```python
from build123d import *

# Parameters (mm, degrees)
SKETCH1_W                    = 22
SKETCH1_H                    = 25
SKETCH1_R                    = 1.5
BASE_FLANGE1_DEPTH           = 1.5
EDGE_FLANGE1_STRIP_W         = 7.4732
EDGE_FLANGE1_STRIP_H         = 1.5
EDGE_FLANGE1_STRIP_CUT_DEPTH = 22
EDGE_FLANGE1_DEPTH           = 22
CUT_EXTRUDE1_DEPTH           = 10


# Sheet-metal steps are written as plain solids
with BuildPart() as part:
    # Sketch1 → Base-Flange1 (new body)
    with BuildSketch(Plane.XY):
        with Locations((0.834482759, -7.531034483)):
            Rectangle(SKETCH1_W, SKETCH1_H)
        with Locations((6.834482759, -13.834829283)):
            Circle(SKETCH1_R, mode=Mode.SUBTRACT)
        with Locations((-5.165517241, -13.834829283)):
            Circle(SKETCH1_R, mode=Mode.SUBTRACT)
        with Locations((-3.415517241, -1.662801421)):
            Circle(SKETCH1_R, mode=Mode.SUBTRACT)
        with Locations((4.994482759, -1.662801421)):
            Circle(SKETCH1_R, mode=Mode.SUBTRACT)
    extrude(amount=-BASE_FLANGE1_DEPTH)

    # Edge-Flange1 strip (across the edge) → Edge-Flange1 strip cut (cut)
    with BuildSketch(Plane(origin=(11.834482759, 4.968965517, 0), x_dir=(0, -1, 0), z_dir=(-1, 0, 0))):
        with Locations((-1.5, -0.75)):
            Rectangle(EDGE_FLANGE1_STRIP_W, EDGE_FLANGE1_STRIP_H)
    extrude(amount=EDGE_FLANGE1_STRIP_CUT_DEPTH, mode=Mode.SUBTRACT)

    # Edge-Flange1 section (across the edge) → Edge-Flange1 (add)
    with BuildSketch(Plane(origin=(11.834482759, 4.968965517, 0), x_dir=(0, -1, 0), z_dir=(-1, 0, 0))):
        with BuildLine():
            Line((0, 0.7366), (0, 14))
            Line((0, 14), (1.5, 14))
            Line((1.5, 14), (1.5, 0.7366))
            ThreePointArc((1.5, 0.7366), (1.715745145, 0.215745145), (2.2366, 0))
            Line((2.2366, 0), (2.2366, -1.5))
            ThreePointArc((2.2366, -1.5), (0.655084973, -0.844915027), (0, 0.7366))
        make_face()
    extrude(amount=EDGE_FLANGE1_DEPTH)

    # Sketch11 → Cut-Extrude1 (cut)
    with BuildSketch(Plane(origin=(0, 4.968965517, 0), x_dir=(1, 0, 0), z_dir=(0, 1, 0))):
        with BuildLine():
            Line((-4.050745128, -10.789495208), (-4.050745128, -4.789495208))
            ThreePointArc((-4.050745128, -4.789495208), (-5.800745128, -3.039495208), (-7.550745128, -4.789495208))
            Line((-7.550745128, -4.789495208), (-7.550745128, -10.789495208))
            ThreePointArc((-7.550745128, -10.789495208), (-5.800745128, -12.539495208), (-4.050745128, -10.789495208))
        make_face()
        with BuildLine():
            Line((8.840531004, -10.789495208), (8.840531004, -4.789495208))
            ThreePointArc((8.840531004, -4.789495208), (7.090531004, -3.039495208), (5.340531004, -4.789495208))
            Line((5.340531004, -4.789495208), (5.340531004, -10.789495208))
            ThreePointArc((5.340531004, -10.789495208), (7.090531004, -12.539495208), (8.840531004, -10.789495208))
        make_face()
    extrude(amount=-CUT_EXTRUDE1_DEPTH, mode=Mode.SUBTRACT)


solid = part.part
```
Could you check a few things on this model? Use its own coordinates, in mm. A direction names the side the tool comes from. Round coordinates to 2 decimals unless told otherwise and drop trailing zeros. Order: outer loops, then holes, each group sorted by start corner. A loop starts at its lowest first (then second) coordinate and runs counter-clockwise, first axis right, second up. Notation, with made-up numbers: M 53,38.25 L 104,38.25 A26 cw 104,59.25 Z; hole C 12.25,56 d3. An arc over 180 degrees is marked long. One line per question, with ' | ' between items. Start each with the question number.
(1) Please list where these lines run through material, in increasing order: line 1 along Z through (x, y) = (3.5, -7.25); line 2 along Y through (x, z) = (10.5, 10.75); line 3 along Z through (x, y) = (8.5, 3.25).
(2) Suppose I cut it at A-A on z = 9.75. List the corners of the cut face in (x, y) for me, then the cut area to 3 significant figures.
(3) Suppose I cut it at C-C on x = 4.5. List the corners of the cut face in (y, z) for me, then the cut area to 3 significant figures.
(4) For P1, Ø6.5, axis at x = -3.5, z = 8.5, coming from the -Y side; P2, Ø10, axis at x = -3.5, y = -2.5, coming from the -Z side; P3, Ø10, axis at x = -7, y = -5.5, coming from the +Z side, each with a flat end and sliding along its axis, tell me the tip position at first contact or that it passes through.
(5) For faces 4 (the face through (-5.76, 4.23, 3.04)), 5 (the face through (1, -8, 0)), 6 (the face through (0.99, 4.3, -0.86)), which set-ups out of +Z, -Z, +X, -X, +Y, -Y let a thin tool reach every point of the face, with its end or its side?
(6) Suppose I cut it at B-B on y = -0.5. List the corners of the cut face in (x, z) for me, then the cut area to 3 significant figures.
(7) Thinking about a two-plate mould opening in Y: for faces 1 (the face through (7.64, -12.57, -0.74)), 2 (the face through (1, -20.031, -1)), 3 (the face through (1, 4.969, 7)), which applies, +Y half, -Y half, draft (parallel to the pull), parting line (faces both ways), or undercut?
(8) Suppose I cut it at D-D on x = -1.25. List the corners of the cut face in (y, z) for me.
Geometry results:
1) line 1: -1.5 to 0 | line 2: 3.47 to 4.97 | line 3: -1.44 to 0.21
2) outline: M -10.17,3.47 L -7.55,3.47 L -7.55,4.97 L -10.17,4.97 Z; M -4.05,3.47 L 5.34,3.47 L 5.34,4.97 L -4.05,4.97 Z; M 8.84,3.47 L 11.83,3.47 L 11.83,4.97 L 8.84,4.97 Z | area: 22.5 mm²
3) outline: M -20.03,-1.5 L -3.08,-1.5 L -3.08,0 L -20.03,0 Z; M -0.25,-1.5 L 2.73,-1.5 A2.24 ccw 4.97,0.74 L 4.97,14 L 3.47,14 L 3.47,0.74 A0.74 cw 2.73,0 L -0.25,0 Z | area: 53.3 mm²
4) P1: y = 3.47 | P2: z = -1.5 | P3: z = 0
5) face 4: +Y, -Y | face 5: +Z, +X, -X, -Y | face 6: -Z, +X, -X, +Y
6) outline: M -10.17,-1.5 L -4.36,-1.5 L -4.36,0 L -10.17,0 Z; M -2.47,-1.5 L 4.05,-1.5 L 4.05,0 L -2.47,0 Z; M 5.94,-1.5 L 11.83,-1.5 L 11.83,0 L 5.94,0 Z | area: 27.3 mm²
7) face 1: undercut | face 2: -Y half | face 3: +Y half
8) outline: M -20.03,-1.5 L 2.73,-1.5 A2.24 ccw 4.97,0.74 L 4.97,14 L 3.47,14 L 3.47,0.74 A0.74 cw 2.73,0 L -20.03,0 Z
